Build history of the part. All positions in model axes, mm. A direction names the side the tool comes from. Give positions to 0.01 mm unless a question says otherwise; leave off trailing zeros. Order: outer loops, then holes, each group sorted by start corner. A loop starts at its lowest first (then second) coordinate and runs counter-clockwise, first axis right, second up. Notation, with made-up numbers: (-5.75, 59.5) - (26.25, 59.5) arc R32 cw to (26.25, 91.5) - close; hole circle Ø1 at (53.25, 16.25). An arc over 180 degrees is marked (long way). Use a Markdown table: item, result. Add a question column.
(1) Slice it at C-C (y = 1.75). Write the cut outline in (x, z) (3 decimals), then the cut area to 3 significant figures.
(2) Slice it at A-A (z = 19.52). Write the cut outline in (x, y).
(3) Slice it at D-D (x = 4.1). Count the separate pieces of the cut face and the enclosed holes in it, then the cut area to 3 significant figures.
(4) Mould opens along Y. For faces 1 (the face through (4.122, 21.913, 21.217)), 2 (the face through (2.05, 9, 8)), 3 (the face through (2.7, 22.55, 20.4)) say: +Y half, -Y half, draft (parallel to the pull), parting line (faces both ways), or undercut.
(5) Slice it at B-B (y = 16.5). Write the cut outline in (x, z) (3 decimals).
(6) Flat gauge pins, fed straight in: pin 1 (2 mm diameter, centred on x = 3, y = 16.5, fed in from -Z) (3 decimals); pin 2 (0.5 mm diameter, centred on y = -0.5, z = -2.5, fed in from -X) (3 decimals); pin 3 (1.3 mm diameter, centred on x = 4.5, z = 3, fed in from +Y). Where does each tip first touch, or does it go through?
(7) Wall check: line 1 (Z direction, x = 4.1, y = 2.5) (3 decimals); line 2 (Y direction, x = 4.85, z = -0.5); line 3 (Z direction, x = 5, y = 11.75) (3 decimals). Give the ranges that are in metal, low to high.
(8) Which spindle directions (+Z, -Z, +X, -X, +Y, -Y) get a long thin tool onto all of the face, cutting with end or side? Do faces 4 (the face through (5.1, 19, 21)), 5 (the face through (2.6, 17.6, 19.5)), 6 (the face through (4, 3, 4.575)). Say none if no direction does.
Autodesk Inventor part; units mm, degrees
ref_plane "YZ Plane" through (0, 0, 0) normal (1, 0, 0) x (0, 1, 0)
ref_plane "XZ Plane" through (0, 0, 0) normal (0, 1, 0) x (-1, 0, 0)
ref_plane "XY Plane" through (0, 0, 0) normal (0, 0, 1) x (1, 0, 0)
sketch "Sketch1" plane through (0, 0, 0) normal (0, 1, 0) x (-1, 0, 0)
  line L0 (-2.05, -5.575) -> (-6.15, -5.575)
  line L1 (-6.15, -5.575) -> (-6.15, 4.575)
  line L2 (-6.15, 4.575) -> (-2.05, 4.575)
  line L3 (-2.05, 4.575) -> (-2.05, -5.575)
  line L4 (-3.175, 4.575) -> (-5.025, 4.575)
  line L5 (-3.175, 4.575) -> (-3.175, -5.575)
  line L6 (-5.025, 4.575) -> (-5.025, -5.575)
  circle A0 centre (-4.1, 3.075) radius 0.75
  circle A1 centre (-4.1, -4.075) radius 0.75
  point P0 (-4.1, 4.575)
  point P1 (-4.1, -5.575)
  point P2 (-1.1679, -0.0702)
  point P3 (-4.1, 4.575)
  dimension "d13" = 4.1
  dimension "d14" = 10.15
  dimension "d44" = 1.85
  dimension "d45" = 1.125
  dimension "d46" = 1.5
  dimension "d47" = 1.5
  dimension "d48" = 1.5
  dimension "d49" = 1.5
extrude "Extrusion1" add sketch "Sketch1" along normal blind 10.15
sketch "Sketch11" plane through (2.05, 0, 4.575) normal (0, 0, 1) x (1, 0, 0)
  point P0 (-2.05, 0)
extrude "Extrusion6" add sketch "Sketch1" against normal blind 1 contours L0 L6 L2 L5
sketch "Sketch12" plane through (0, 10.15, 0) normal (0, 1, 0) x (1, 0, 0)
  circle A0 centre (4.0754, 4.0842) radius 1.265
  circle A1 centre (4.0754, -3.0807) radius 1.265
  point P0 (0, 0)
  dimension "d52" = 2.53
  dimension "d53" = 2.53
extrude "Extrusion7" cut sketch "Sketch12" against normal blind 1
sketch "Sketch13" plane through (2.05, 10.15, 4.575) normal (0, 0, 1) x (1, 0, 0)
  line L0 (0, 0) -> (0, -4.15)
  line L1 (0, -10.15) -> (0, 0)
  line L2 (0, -4.15) -> (4.1, -4.15)
  line L3 (4.1, -10.15) -> (4.1, 0)
  line L4 (4.1, 0) -> (4.1, -4.15)
  line L5 (0, 0) -> (4.1, 0)
  point P0 (-2.05, -10.15)
  dimension "d56" = 4.15
extrude "Extrusion8" add sketch "Sketch13" along normal blind 17
sketch "Sketch14" plane through (0, 10.15, 0) normal (0, 1, 0) x (1, 0, 0)
  line L0 (6.15, 5.575) -> (6.15, -21.575)
  line L1 (6.15, -21.575) -> (6.15, -17.465)
  line L2 (6.15, -17.465) -> (2.05, -17.465)
  line L3 (2.05, 5.575) -> (2.05, -21.575)
  line L4 (2.05, -21.575) -> (6.15, -21.575)
  point P0 (0, 0)
  dimension "d59" = 4.11
extrude "Extrusion9" add sketch "Sketch14" along normal blind 12.4
sketch "Sketch15" plane through (2.05, 10.15, 21.575) normal (0, 0, 1) x (1, 0, 0)
  line L0 (2.05, 10.7632) -> (2.05, 7.9632) construction
  line L1 (4.1, 0) -> (4.1, 12.4)
  line L2 (1.05, 10.7632) -> (1.05, 7.9632)
  line L3 (3.05, 7.9632) -> (3.05, 10.7632)
  arc A0 (3.05, 10.7632) -> (1.05, 10.7632) centre (2.05, 10.7632) ccw
  arc A1 (1.05, 7.9632) -> (3.05, 7.9632) centre (2.05, 7.9632) ccw
  point P0 (-2.05, -10.15)
  point P1 (2.05, 9.3632)
  dimension "d62" = 1.4
  dimension "d63" = 2
  dimension "d64" = 2.05
extrude "Extrusion10" cut sketch "Sketch15" against normal through all
sketch "Sketch16" plane through (0, 22.55, 0) normal (0, 1, 0) x (1, 0, 0)
  circle A0 centre (4.1, -19.52) radius 1.5
  line L0 (2.05, -21.575) -> (6.15, -21.575)
  line L1 (6.15, -21.575) -> (6.15, -17.465)
  point P0 (0, 0)
  point P1 (4.1, -21.575)
  dimension "d67" = 3
  dimension "d68" = 2.055
  dimension "d69" = 2.05
extrude "Extrusion11" cut sketch "Sketch16" against normal blind 10
equation "\"d13\" = base_width"
equation "\"d45\" = -0.5 * d44 + 0.5 * d13"
equation "\"d4\" = base_length"
equation "\"base_width\" = 4.1"
equation "\"base_length\" = 10.15"
equation "\"base_screw_diameter\" = 1.5"
equation "\"base_screw_spacing_edge\" = 8.5"
properties part number "original_holder"
Solution:
| question | item | result |
|---|---|---|
| 1 | outline | (2.05, -5.575) - (6.15, -5.575) - (6.15, 4.575) - (2.05, 4.575) - close; hole circle Ø1.5 at (4.1, -4.075); hole circle Ø1.5 at (4.1, 3.075) |
| 1 | area | 38.1 mm2 |
| 2 | outline | (2.05, 6) - (6.15, 6) - (6.15, 22.55) - (5.6, 22.55) - (5.6, 12.55) - (2.6, 12.55) - (2.6, 22.55) - (2.05, 22.55) - close |
| 3 | separate pieces | 5 |
| 3 | enclosed holes | 0 |
| 3 | area | 164 mm2 |
| 4 | face 1 | undercut |
| 4 | face 2 | draft |
| 4 | face 3 | +Y half |
| 5 | outline | (2.05, 17.465) - (6.15, 17.465) - (6.15, 21.575) - (2.05, 21.575) - close; hole circle Ø3 at (4.1, 19.52) |
| 6 | pin 1 | z = 17.465 |
| 6 | pin 2 | x = 3.175 |
| 6 | pin 3 | y = 9.15 |
| 7 | line 1 | -5.575 to -4.825, -3.325 to 2.325, 3.825 to 4.575 |
| 7 | line 2 | -1 to 10.15 |
| 7 | line 3 | 17.465 to 21.575 |
| 8 | face 4 | +Z, -Z |
| 8 | face 5 | +Y |
| 8 | face 6 | +Z, +X, -X, -Y |
